Can you work these out from the drawing? Everything is in mm from the part's minimum corner. A direction names the side the tool comes from. Give positions to 0.01 mm unless a question says otherwise; leave off trailing zeros. Write each loop counter-clockwise with the first axis right and the second up, starting at its lowest first coordinate (ties: lowest second). Pieces come first, ordered by that corner, then holes. Notation, with made-up numbers: (54, -9) - (112, -9) arc R19 ccw to (112, 8) - close; hole circle Ø11 at (66.25, 73.5). An arc over 180 degrees is marked (long way). Use a Markdown table: item, result.
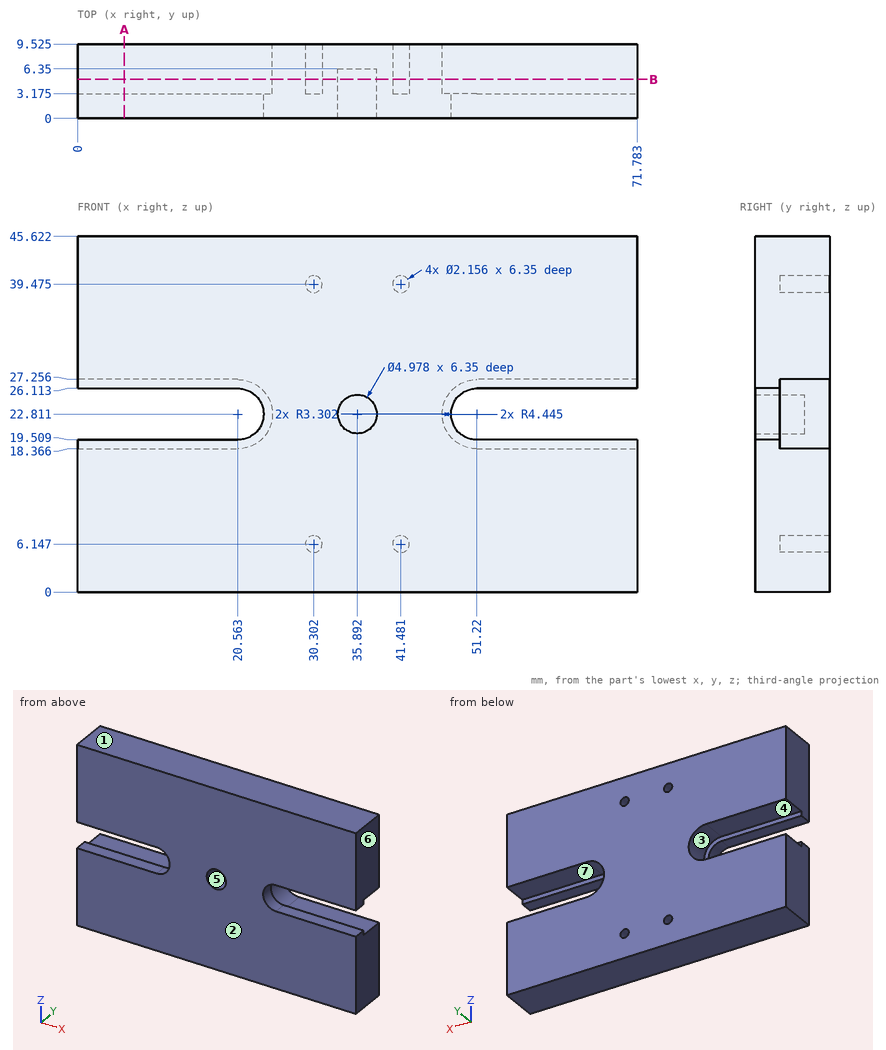
Item 1: For the marked faces 4, 5, 6 and 7, which set-ups out of +Z, -Z, +X, -X, +Y, -Y let a thin tool reach every point of the face, with its end or its side?
Values:
| item | result |
|---|---|
| face 4 | -X, +Y |
| face 5 | -Y |
| face 6 | +Z, -Z, +X, +Y, -Y |
| face 7 | +X, +Y |
Item 2: Will these pins go through, and if not, where does the flat tip stop? pin 1 Ø0.6 at (x, z) = (30.5, 6) entering from +Y (1 decimal); pin 2 Ø4.5 at (x, z) = (35.89, 22.81) entering from -Y.
Values:
| item | result |
|---|---|
| pin 1 | stops at y = 3.2 |
| pin 2 | stops at y = 6.35 |
Item 3: Thinking about a two-plate mould opening in Z: for the marked faces 1, 2 and 3, which applies, +Z half, -Z half, draft (parallel to the pull), parting line (faces both ways), or undercut?
Values:
| item | result |
|---|---|
| face 1 | +Z half |
| face 2 | draft |
| face 3 | undercut |
Item 4: I need wall thicknesses on line 1 along Z through (x, y) = (59, 4.75) (1 decimal); line 2 along Z through (x, y) = (11, 2); line 3 along X through (y, z) = (6.75, 38.5) (1 decimal). Which ranges of each line are inside material? Lowest first, please. Write a range as [from, to].
Values:
| item | result |
|---|---|
| line 1 | z = [0, 18.4], [27.3, 45.6] |
| line 2 | z = [0, 19.51], [26.11, 45.62] |
| line 3 | x = [0, 29.8], [30.8, 41], [41.9, 71.8] |
Item 5: If we section it at B-B, the plane y = 5: Write out the boundary of the cut face in (x, z) (1 decimal), plus the area to 3 significant figures.
Values:
| item | result |
|---|---|
| outline | (0, 0) - (71.8, 0) - (71.8, 18.4) - (51.2, 18.4) arc R4.4 cw to (51.2, 27.3) - (71.8, 27.3) - (71.8, 45.6) - (0, 45.6) - (0, 27.3) - (20.6, 27.3) arc R4.4 cw to (20.6, 18.4) - (0, 18.4) - close; hole circle Ø2.2 at (30.3, 6.1); hole circle Ø2.2 at (30.3, 39.5); hole circle Ø5 at (35.9, 22.8); hole circle Ø2.2 at (41.5, 6.1); hole circle Ø2.2 at (41.5, 39.5) |
| area | 2,810 mm2 |
Item 6: If we section it at A-A, the plane x = 6: Write out the boundary of the cut face in (y, z) (1 decimal), plus the area to 3 significant figures.
Values:
| item | result |
|---|---|
| outline | (0, 0) - (9.5, 0) - (9.5, 18.4) - (3.2, 18.4) - (3.2, 19.5) - (0, 19.5) - close; (0, 26.1) - (3.2, 26.1) - (3.2, 27.3) - (9.5, 27.3) - (9.5, 45.6) - (0, 45.6) - close |
| area | 357 mm2 |
